Verification items for the finished model (mm, model axes). A direction names the side the tool comes from. Coordinates: 2 decimals unless noted, no trailing zeros. Order: outer loops, then holes, each group sorted by start corner. A loop starts at its lowest first (then second) coordinate and runs counter-clockwise, first axis right, second up. Notation, with made-up numbers: (73, -30) -> (104, -30) arc R9 ccw to (104, -13) -> close; hole circle Ø10 at (-25, 28.5). An arc over 180 degrees is marked (long way). Answer as CSV lines item,"result".
```python
from build123d import *

# Parameters (mm, degrees)
SKETCH2_R                = 5.500000001
BOSS_EXTRUDE2_DEPTH      = 3.5
SKETCH3_R                = 7.000000001
BOSS_EXTRUDE3_DEPTH      = 3
CHAMFER1_SIZE            = 1
CHAMFER1_OF_MIRROR1_SIZE = 1
CUT_EXTRUDE1_DEPTH       = 12.842719284
CUT_EXTRUDE1_DEPTH_BACK  = 12.842719284
SKETCH4_R                = 2.5
CHAMFER2_SIZE            = 0.25


with BuildPart() as part:
    # Sketch2 → Boss-Extrude2 (new, symmetric)
    with BuildSketch(Plane.XZ):
        with Locations(Location((0, 0, 0), (0, 0, 270))):
            Circle(SKETCH2_R)
    extrude(amount=BOSS_EXTRUDE2_DEPTH, both=True)

    # Sketch3 → Boss-Extrude3 (add)
    with BuildSketch(Plane(origin=(0, -3.5, 0), x_dir=(1, 0, 0), z_dir=(0, 1, 0))):
        with Locations(Location((0, 0, 0), (0, 0, 90))):
            Circle(SKETCH3_R)
    boss_extrude3 = extrude(amount=-BOSS_EXTRUDE3_DEPTH)

    # Chamfer1
    chamfer1_edges = [part.edges().sort_by_distance(p)[0] for p in [
        (0, -6.5, 7.000000001),
    ]]
    chamfer(chamfer1_edges, length=CHAMFER1_SIZE)

    # Mirror1: Boss-Extrude3 across plane
    add(boss_extrude3.mirror(Plane.ZX))

    # Chamfer1 of Mirror1
    chamfer1_of_mirror1_edges = [part.edges().sort_by_distance(p)[0] for p in [
        (0, 6.5, 7.000000001),
    ]]
    chamfer(chamfer1_of_mirror1_edges, length=CHAMFER1_OF_MIRROR1_SIZE)

    # Sketch4 → Cut-Extrude1 (cut, two sides: drawn at the far end of the back side and taken through both)
    with BuildSketch(Plane(origin=(0, 0, 0), x_dir=(-1, 0, 0), z_dir=(0, 1, 0)).offset(-CUT_EXTRUDE1_DEPTH_BACK)):
        with Locations(Location((0, 0, 0), (0, 0, 270))):
            Circle(SKETCH4_R)
    extrude(amount=CUT_EXTRUDE1_DEPTH + CUT_EXTRUDE1_DEPTH_BACK, mode=Mode.SUBTRACT)

    # Chamfer2
    chamfer2_edges = [part.edges().sort_by_distance(p)[0] for p in [
        (0, -6.5, 2.5),
        (0, 6.5, 2.5),
    ]]
    chamfer(chamfer2_edges, length=CHAMFER2_SIZE)


solid = part.part
```
Item 1: Section check A-A, the plane x = 0. Record the boundary of the cut face in (y, z), plus the area to 3 significant figures.
Answer list:
outline,"(-6.5, -6) -> (-5.5, -7) -> (-3.5, -7) -> (-3.5, -5.5) -> (3.5, -5.5) -> (3.5, -7) -> (5.5, -7) -> (6.5, -6) -> (6.5, -2.75) -> (6.25, -2.5) -> (-6.25, -2.5) -> (-6.5, -2.75) -> close; (-6.5, 2.75) -> (-6.25, 2.5) -> (6.25, 2.5) -> (6.5, 2.75) -> (6.5, 6) -> (5.5, 7) -> (3.5, 7) -> (3.5, 5.5) -> (-3.5, 5.5) -> (-3.5, 7) -> (-5.5, 7) -> (-6.5, 6) -> close"
area,"93.9 mm2"
Item 2: Thickness scan on line 1 (Y direction, x = 3.5, z = -4.5); line 2 (X direction, y = -1, z = 0); line 3 (Y direction, x = -4.5, z = 4.75). Record the ranges inside material, lowest first.
Answer list:
line 1,"-6.5 to -3.5, 3.5 to 6.5"
line 2,"-5.5 to -2.5, 2.5 to 5.5"
line 3,"-5.96 to -3.5, 3.5 to 5.96"
Item 3: Depth check by flat-ended pin: pin 1 Ø1.5 at (x, y) = (3.5, 2.5) entering from +Z; pin 2 Ø5 at (x, y) = (3, -4.5) entering from -Z. Enter the tip coordinate at first touch or a pass-through.
Answer list:
pin 1,"z = 4.76"
pin 2,"z = -6.98"
Item 4: Tool access check on faces 5 (the flat face through (4, -3.5, 4)), 6 (the cylindrical face through (4.259, -4.486, 5.555)). Record the directions out of +Z, -Z, +X, -X, +Y, -Y that give a thin tool (end or side, any length) a straight path to the whole face; none if there is none.
Answer list:
face 5,"none"
face 6,"+Y, -Y"
Item 5: Section check D-D, the plane y = 5.25. Record the boundary of the cut face in (x, z), plus the area to 3 significant figures.
Answer list:
outline,"circle Ø14 at (0, 0); hole circle Ø5 at (0, 0)"
area,"134 mm2"
Item 6: Section check B-B, the plane z = 0. Record the boundary of the cut face in (x, y).
Answer list:
outline,"(-7, -5.5) -> (-6, -6.5) -> (-2.75, -6.5) -> (-2.5, -6.25) -> (-2.5, 6.25) -> (-2.75, 6.5) -> (-6, 6.5) -> (-7, 5.5) -> (-7, 3.5) -> (-5.5, 3.5) -> (-5.5, -3.5) -> (-7, -3.5) -> close; (2.5, -6.25) -> (2.75, -6.5) -> (6, -6.5) -> (7, -5.5) -> (7, -3.5) -> (5.5, -3.5) -> (5.5, 3.5) -> (7, 3.5) -> (7, 5.5) -> (6, 6.5) -> (2.75, 6.5) -> (2.5, 6.25) -> close"
Item 7: Release check for a two-part mould opening along Y. For faces 1 (the cylindrical face through (-5.37, -0.05, 1.19)), 2 (the flat face through (1, 6.5, -3)), 3 (the flat face through (1, -6.5, -3)), 4 (the cylindrical face through (2.44, -0.09, 0.54)) record: +Y half, -Y half, draft (parallel to the pull), parting line (faces both ways), or undercut.
Answer list:
face 1,"undercut"
face 2,"+Y half"
face 3,"-Y half"
face 4,"draft"
Item 8: Section check C-C, the plane y = 0. Record the boundary of the cut face in (x, z), plus the area to 3 significant figures.
Answer list:
outline,"circle Ø11 at (0, 0); hole circle Ø5 at (0, 0)"
area,"75.4 mm2"
